Autodesk Inventor part; units mm, degrees
ref_plane "Work Plane1" through (0, 0, -15) normal (0, 0, 1) x (1, 0, 0)
ref_plane "YZ Plane" through (0, 0, 0) normal (1, 0, 0) x (0, 1, 0)
ref_plane "XZ Plane" through (0, 0, 0) normal (0, 1, 0) x (-1, 0, 0)
sketch "Sketch1" plane through (0, 0, 0) normal (0, 0, 1) x (1, 0, 0)
  line L0 (0, 0) -> (25, 0)
  line L1 (25, 0) -> (25, 40)
  line L2 (25, 40) -> (0, 40)
  line L3 (0, 40) -> (0, 0)
  dimension "d1" = 25
  dimension "d2" = 40
  dimension "d3" = 25
extrude "Extrusion1" add sketch "Sketch1" against normal blind 30
sketch "Sketch2" plane through (25, 0, 0) normal (1, 0, 0) x (0, 0, -1)
  line L0 (0, 0) -> (30, 0)
  circle A0 centre (15, 6.56) radius 2.46
extrude "Extrusion2" cut sketch "Sketch2" against normal blind 30
sketch "Sketch3" plane through (0, 0, 0) normal (-1, 0, 0) x (0, 0, 1)
  line L0 (0, 0) -> (-30, 0)
  line L1 (-25.05, 0) -> (-4.95, 0)
  line L2 (-4.95, 0) -> (-4.95, 33.12)
  line L3 (-4.95, 33.12) -> (-25.05, 33.12)
  line L4 (-25.05, 33.12) -> (-25.05, 0)
  dimension "d11" = 20.1
extrude "Extrusion3" cut sketch "Sketch3" against normal blind 20
sketch "Sketch4" plane through (0, 0, 0) normal (0, -1, 0) x (1, 0, 0)
  line L0 (20, -4.95) -> (20, -25.05)
  line L1 (20, -15) -> (25, -15)
  line L2 (25, 0) -> (25, -30)
  line L3 (20, -8.025) -> (25, -8.025)
  line L4 (25, -8.025) -> (25, -21.975)
  line L5 (25, -21.975) -> (20, -21.975)
  line L6 (20, -21.975) -> (20, -8.025)
  line L7 (20, -8.025) -> (25, -21.975) construction
  line L8 (25, -8.025) -> (20, -21.975) construction
  line L9 (25, -12.54) -> (25, -17.46)
  point P0 (0, 0)
  point P1 (22.5, -15)
  dimension "d14" = 13.95
extrude "Extrusion4" add sketch "Sketch4" along normal blind 15
sketch "Sketch5" plane through (20, 0, 0) normal (-1, 0, 0) x (0, 0, 1)
  circle A0 centre (-15, 6.56) radius 2.46
  circle A1 centre (-15, 6.56) radius 4.7025
  circle A2 centre (-15, 6.56) radius 2.46
  circle A3 centre (-15, 6.56) radius 2.46
  point P0 (0, 0)
  dimension "d17" = 9.405
extrude "Extrusion5" cut sketch "Sketch5" against normal blind 2.1
sketch "Sketch6" plane through (25, 0, 0) normal (1, 0, 0) x (0, 0, -1)
  circle A0 centre (15, 6.56) radius 4.7025
  line L0 (15, 6.56) -> (15, 23.56)
  circle A1 centre (15, 23.56) radius 2.46
  point P0 (0, 0)
  dimension "d20" = 17
  dimension "d21" = 4.92
extrude "Extrusion6" cut sketch "Sketch6" against normal blind 10 contours A1
sketch "Sketch7" plane through (20, 0, 0) normal (-1, 0, 0) x (0, 0, 1)
  circle A0 centre (-15, 23.56) radius 2.46
  circle A1 centre (-15, 23.56) radius 4.7025
  point P0 (0, 0)
  dimension "d24" = 9.405
extrude "Extrusion7" cut sketch "Sketch7" against normal blind 2.1
sketch "Sketch9" plane through (25, 0, 0) normal (1, 0, 0) x (0, 0, -1)
  circle A0 centre (15, 6.56) radius 2.46
  circle A1 centre (15, 6.56) radius 2.46
  circle A2 centre (15, 23.56) radius 2.46
  circle A3 centre (15, 23.56) radius 2.46
  line L0 (30, 40) -> (30, 0)
  line L1 (30, 0) -> (30, 40)
  line L2 (30, 40) -> (0, 40)
  line L3 (0, 40) -> (0, 0)
  line L4 (0, 0) -> (8.025, 0)
  line L5 (21.975, 0) -> (21.975, -15)
  line L6 (21.975, -15) -> (8.025, -15)
  line L7 (8.025, -15) -> (8.025, 0)
  line L8 (0, 0) -> (8.025, 0)
  line L9 (21.975, 0) -> (30, 0)
extrude "Extrusion8" add sketch "Sketch9" along normal blind 5
sketch "Sketch10" plane through (0, 40, 0) normal (0, 1, 0) x (1, 0, 0)
  line L0 (0, 30) -> (30, 30)
  line L1 (30, 0) -> (0, 0)
  line L2 (0, 30) -> (30, 30)
  line L3 (30, 30) -> (30, 0)
  line L4 (30, 0) -> (0, 0)
  line L5 (0, 0) -> (0, 30)
extrude "Extrusion9" add sketch "Sketch10" along normal blind 30
sketch "Sketch12" plane through (30, 0, 0) normal (1, 0, 0) x (0, 0, -1)
  circle A0 centre (15, 6.56) radius 2.46
  line L0 (15, 6.56) -> (15, 15.06)
  circle A1 centre (15, 15.06) radius 2.525
  point P0 (0, 0)
  dimension "d31" = 8.5
  dimension "d33" = 5.05
extrude "Extrusion10" cut sketch "Sketch12" against normal blind 30 contours A1
sketch "Sketch15" plane through (0, 0, -25.05) normal (-1, 0, 0) x (0, 0, 1)
  line L0 (0, 33.12) -> (20.1, 33.12)
  line L1 (20.1, 33.12) -> (20.1, 0)
  line L2 (0, 33.12) -> (20.1, 33.12)
  line L3 (20.1, 33.12) -> (20.1, 31.1)
  line L4 (20.1, 31.1) -> (0, 31.1)
  line L5 (0, 31.1) -> (0, 33.12)
  point P0 (25.05, 0)
  dimension "d57" = 2.02
extrude "Extrusion13" add sketch "Sketch15" against normal blind 20
sketch "Sketch17" plane through (0, 0, 0) normal (0, 0, 1) x (1, 0, 0)
  line L0 (0, 70) -> (30, 70)
  line L1 (30, 70) -> (50.0622, 90.0622)
  line L2 (30, 70) -> (80, 70) construction
  line L3 (11.9522, 97.2454) -> (0, 85.2932)
  line L4 (0, 70) -> (0, 85.2932)
  line L5 (0, 70) -> (0, 0)
  line L6 (0, 70) -> (30, 70)
  line L7 (10.923, 112.2849) -> (0, 120.567)
  line L8 (50.0622, 105.3553) -> (50.0622, 120.567)
  line L9 (50.0622, 105.3553) -> (50.0622, 90.0622)
  arc A0 (11.9522, 97.2454) -> (10.923, 112.2849) centre (4.8811, 104.3165) ccw
  line L10 (0, 165.567) -> (30, 165.567)
  line L11 (30, 165.567) -> (50.0622, 120.567)
  line L12 (6, 163.067) -> (0, 165.567)
  line L13 (6, 123.067) -> (0, 120.567)
  line L14 (6, 123.067) -> (12, 143.067)
  line L15 (12, 143.067) -> (6, 163.067)
  dimension "d61" = 45
  dimension "d62" = 32.0271
  dimension "d72" = 10
extrude "Extrusion14" add sketch "Sketch17" against normal blind 30
sketch "Sketch24" plane through (0, 0, 0) normal (0, 0, 1) x (1, 0, 0)
  line L0 (30, 70) -> (50.0622, 90.0622)
  line L1 (30, 70) -> (50.0622, 90.0622)
  line L2 (50.0622, 90.0622) -> (50.0622, 120.567)
  line L3 (50.0622, 90.0622) -> (50.0622, 120.567)
  line L4 (30, 165.567) -> (50.0622, 120.567)
  line L5 (50.0622, 120.567) -> (30, 165.567)
  line L6 (0, 165.567) -> (30, 165.567)
  line L7 (30, 165.567) -> (0, 165.567)
  line L8 (6, 163.067) -> (0, 165.567)
  line L9 (0, 165.567) -> (6, 163.067)
  line L10 (12, 143.067) -> (6, 163.067)
  line L11 (6, 163.067) -> (12, 143.067)
  line L12 (6, 123.067) -> (12, 143.067)
  line L13 (12, 143.067) -> (6, 123.067)
  line L14 (0, 120.567) -> (6, 123.067)
  line L15 (6, 123.067) -> (0, 120.567)
  line L16 (10.923, 112.2849) -> (0, 120.567)
  line L17 (0, 120.567) -> (10.923, 112.2849)
  line L18 (0, 85.2932) -> (11.9522, 97.2454)
  line L19 (11.9522, 97.2454) -> (0, 85.2932)
  line L20 (0, 85.2932) -> (0, 55.2932)
  line L21 (0, 0) -> (0, 85.2932)
  line L22 (0, 55.2932) -> (30, 55.2932)
  line L23 (30, 0) -> (30, 70)
  line L24 (30, 55.2932) -> (30, 70)
  arc A0 (11.9522, 97.2454) -> (10.923, 112.2849) centre (4.8811, 104.3165) ccw
  arc A1 (11.9522, 97.2454) -> (10.923, 112.2849) centre (4.8811, 104.3165) ccw
  dimension "d102" = 30
extrude "Extrusion15" add sketch "Sketch24" along normal blind 30
ref_plane "Work Plane1" through (0, 0, -15) normal (0, 0, 1) x (1, 0, 0)
mirror "Mirror1" about plane through (0, 0, -15) normal (0, 0, 1) of "Extrusion15"
properties part number "rec_c_40mm_x_90mm"
The model under review builds one solid part; all positions refer to its coordinate system, in mm. A direction names the side the tool comes from. Give positions to 0.01 mm unless a question says otherwise; leave off trailing zeros. Write each loop counter-clockwise with the first axis right and the second up, starting at its lowest first coordinate (ties: lowest second). Pieces come first, ordered by that corner, then holes. Notation, with made-up numbers: (76.5, 40.5) -> (92.5, 40.5) arc R18 cw to (92.5, 74.5) -> close; hole circle Ø10 at (6.5, -6). An arc over 180 degrees is marked (long way). Put each result on its own line as item: value.
(1) We need section C-C, the plane z = 5.5. Give the boundary of the cut face in (x, y).
Results are:
outline: (0, 55.29) -> (30, 55.29) -> (30, 70) -> (50.06, 90.06) -> (50.06, 120.57) -> (30, 165.57) -> (0, 165.57) -> (6, 163.07) -> (12, 143.07) -> (6, 123.07) -> (0, 120.57) -> (10.92, 112.28) arc R10 cw to (11.95, 97.25) -> (0, 85.29) -> close
(2) We need section A-A, the plane x = 24.5. Give the boundary of the cut face in (y, z) (3 decimals).
Results are:
outline: (-15, -21.975) -> (0, -21.975) -> (0, -30) -> (55.293, -30) -> (55.293, -60) -> (165.567, -60) -> (165.567, 30) -> (55.293, 30) -> (55.293, 0) -> (0, 0) -> (0, -8.025) -> (-15, -8.025) -> close; hole circle Ø4.92 at (6.56, -15); hole circle Ø5.05 at (15.06, -15); hole circle Ø4.92 at (23.56, -15)
(3) For pin 1 Ø6 at (y, z) = (12.5, -12.5) entering from -X; pin 2 Ø6 at (x, y) = (10, 15.5) entering from +Z; pin 3 Ø15 at (y, z) = (23.56, -15) entering from +X, all flat-tipped, find the tip position at first contact; note any pin that passes through.
Results are:
pin 1: x = 20
pin 2: z = 0
pin 3: x = 30
(4) We need section B-B, the plane y = 15.06. Give the boundary of the cut face in (x, z) (3 decimals), and give its area (4 significant figures).
Results are:
outline: (0, -30) -> (30, -30) -> (30, -17.525) -> (20, -17.525) -> (20, -25.05) -> (0, -25.05) -> close; (0, -4.95) -> (20, -4.95) -> (20, -12.475) -> (30, -12.475) -> (30, 0) -> (0, 0) -> close
area: 447.5 mm²
(5) To check wall thickness, follow probe 1 along Y at (x, z) = (21.2, -15) (1 decimal); probe 2 along Y at (x, z) = (24.75, -15) (3 decimals); probe 3 along Z at (x, y) = (5, 30.5). State the ranges of each line that lie inside material, in increasing order. Write a range as from..to.
Results are:
probe 1: -15..1.9, 11.3..12.5, 17.6..18.9, 28.3..165.6
probe 2: -15..4.1, 9.02..12.535, 17.585..21.1, 26.02..165.567
probe 3: -30..-25.05, -4.95..0
(6) The part is to be moulded in two halves that separate along Z. For faces 5 (the flat face through (25, -15, -15)), 6 (the flat face through (25, -8, -8.025)), 7 (the flat face through (25, 111, -60)), 8 (the flat face through (20, 8, -20)), say which applies: pulls with the +Z half, pulls with the -Z half, needs draft (parallel to the pull), parting line crosses it, or undercut.
Results are:
face 5: needs draft
face 6: pulls with the +Z half
face 7: pulls with the -Z half
face 8: undercut
(7) We need section D-D, the plane z = -15. State how many separate pieces and enclosed holes the cut face has, and give its area (3 significant figures).
Results are:
separate pieces: 4
enclosed holes: 0
area: 4,890 mm²
(8) Tool access review of faces 1 (the flat face through (25, -7, -21.975)), 2 (the flat face through (22.1, 4.5, -13)), 3 (the flat face through (15, 0, -3)), 4 (the flat face through (3.042, 121.835, -14.37)): name each direction out of +Z, -Z, +X, -X, +Y, -Y from which nothing blocks a thin tool from reaching the whole face with its end or side.
Results are:
face 1: -Z, +X, -X, -Y
face 2: -X
face 3: +Z, +X, -X, -Y
face 4: +Z, -Z, -X
